For this review, use the dimensioned drawing (mm, ordinates from the lowest corner) and the shaded views. A direction names the side the tool comes from. Round coordinates to 2 decimals unless told otherwise and drop trailing zeros. Loops run counter-clockwise (first coordinate to the right, second up) from the corner with the lowest first, then second, coordinate; pieces in that order, holes last. Notation, with made-up numbers: (73.25, 53.25) - (111.25, 53.25) arc R28 ccw to (111.25, 84.25) - close; hole circle Ø3 at (74.5, 40.25). An arc over 180 degrees is marked (long way). Use one line per item in the form item = value. Start each with the question number.
(1) For pin 1 (3.5 mm diameter, centred on y = 79, z = 47.5, fed in from +X); pin 2 (1.8 mm diameter, centred on x = 14, z = 49.5, fed in from -Y); pin 3 (11 mm diameter, centred on x = 45, y = 75.5, fed in from -Z), all flat-tipped, find the tip position at first contact; note any pin that passes through.
(2) We need section C-C, the plane x = 23.5. Write out the cut boundary in (y, z) (1 decimal), then the cut area to 3 significant figures.
(3) We need section A-A, the plane z = 50. Write out the cut boundary in (x, y), then the cut area to 3 significant figures.
(4) We need section B-B, the plane y = 8. Write out the cut boundary in (x, z).
(5) Wall thickness on probe 1 along Z at (x, y) = (36.5, 50); probe 2 along X at (y, z) = (10, 34); probe 3 along Z at (x, y) = (23.5, 50): over which ranges is each line inside the solid? List them lowest first. Write a range as [from, to].
(6) Machinability: for the marked faces 4 and 5, which of the approach directions +Z, -Z, +X, -X, +Y, -Y give a long, thin tool a straight path to every point of the face, cutting with its end or side? Answer none if there is none.
(7) The part is to be moulded in two halves that separate along Z. For the marked faces 1, 2 and 3, say which applies: released by +Z, released by -Z, zero draft, split by the parting line, or undercut.
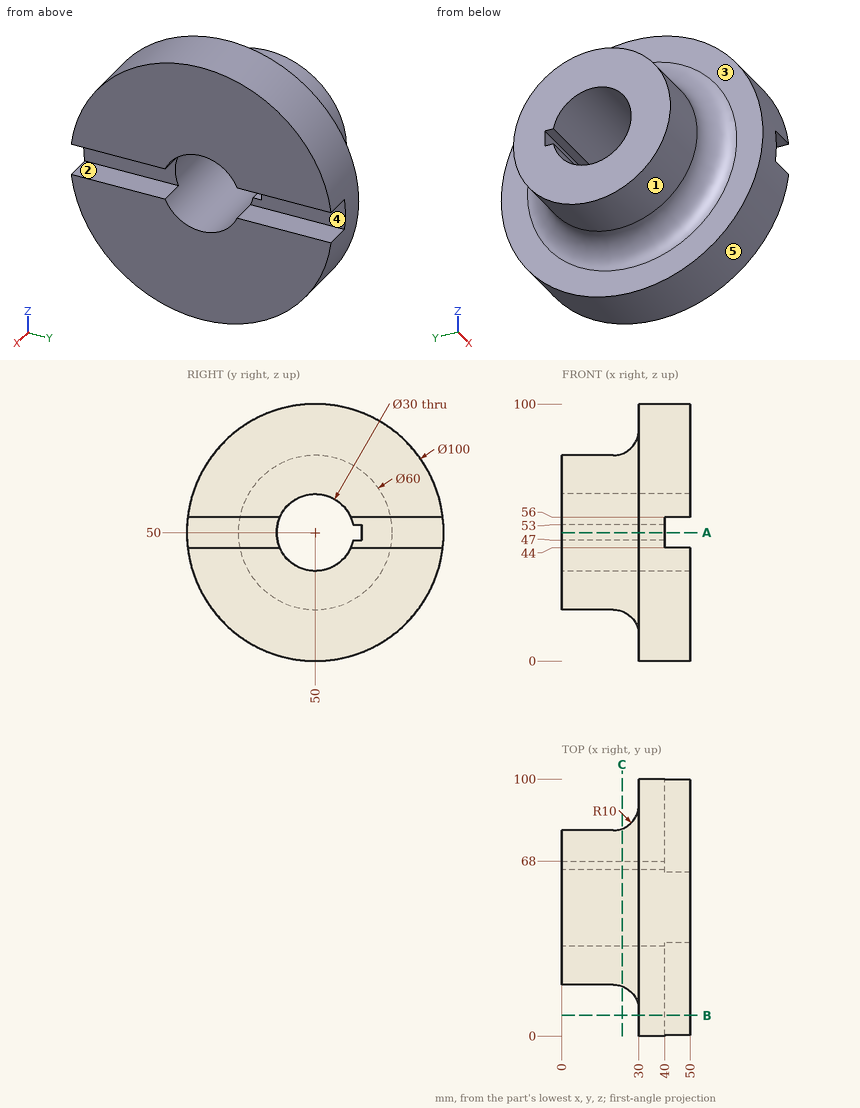
Data:
q1.pin_1 = 40
q1.pin_2 = 20
q1.pin_3 = 4.17
q2.outline = circle Ø61.3 at (50, 50); hole (64.7, 47) - (68, 47) - (68, 53) - (64.7, 53) arc R15 ccw (long way) to start
q2.area = 2,220 mm^2
q3.outline = (0, 20) - (20, 20) arc R10 cw to (30, 10) - (30, 0) - (40, 0) - (40, 35) - (0, 35) - close; (0, 68) - (40, 68) - (40, 100) - (30, 100) - (30, 90) arc R10 cw to (20, 80) - (0, 80) - close
q3.area = 1,520 mm^2
q4.outline = (30, 22.87) - (50, 22.87) - (50, 44) - (40, 44) - (40, 56) - (50, 56) - (50, 77.13) - (30, 77.13) - close
q5.probe_1 = [0, 35], [65, 100]
q5.probe_2 = [30, 50]
q5.probe_3 = [19.37, 35], [65, 80.63]
q6.face_4 = +X, +Y, -Y
q6.face_5 = +X, -X
q7.face_1 = split by the parting line
q7.face_2 = undercut
q7.face_3 = zero draft
